Model file for the job. Use its own axes, mm. A direction names the side the tool comes from. Round coordinates to 2 decimals unless told otherwise and drop trailing zeros. Order: outer loops, then holes, each group sorted by start corner. A loop starts at its lowest first (then second) coordinate and runs counter-clockwise, first axis right, second up. Notation, with made-up numbers: (56, 30.25) -> (107, 30.25) arc R12 cw to (107, 38.25) -> close; hole circle Ø10 at (78.25, 77). An arc over 180 degrees is marked (long way). Answer as CSV lines item,"result".
Solid Edge part; units mm, degrees
sketch "Sketch1" plane through (0, 0, 0) normal (0, 0, 1) x (1, 0, 0)
  line L0 (0, 123.5) -> (0, 6.5)
  line L1 (13, 6.5) -> (13, 123.5)
  arc A0 (13, 6.5) -> (0, 6.5) centre (6.5, 6.5) cw
  arc A1 (0, 123.5) -> (13, 123.5) centre (6.5, 123.5) cw
extrude "Protrusion1" add sketch "Sketch1" along normal blind 6.5
sketch "Sketch2" plane through (6.5, 0, 0) normal (1, 0, 0) x (0, 1, 0)
  line L0 (3.5, 5.5) -> (3.5, 6.5)
  line L1 (3.5, 6.5) -> (6.5, 6.5)
  line L2 (6.5, 1) -> (6.5, 6.5)
  line L3 (3.5, 1) -> (6.5, 1)
  line L4 (3.5, 1) -> (2.6811, 3.25)
  line L5 (3.5, 5.5) -> (2.6811, 3.25)
revolve "RevolvedCutout1" cut sketch "Sketch2" angle 360 about axis through (6.5, 6.5, 1) along (0, 0, 1)
chamfer "Chaflán_38" distance 0.75 angle 45 1 edges at (6.5, 3.5, 6.5)
pattern_linear "Pattern1" count 10 spacing 13 along (0, 1, 0) of "RevolvedCutout1", "Chaflán_38"
chamfer "Chaflán_39" distance 1.5 angle 45 8 edges at (13, 65, 6.5) (6.5, 0, 6.5) (0, 65, 6.5) (6.5, 130, 6.5) (13, 65, 0) (6.5, 0, 0) (0, 65, 0) (6.5, 130, 0)
Q1. Saw through at A-A (y = 78.5). Write the cut outline in (x, z), plus the area to 3 significant figures.
Checks:
outline,"(0, 1.5) -> (1.5, 0) -> (11.5, 0) -> (13, 1.5) -> (13, 5) -> (11.5, 6.5) -> (1.5, 6.5) -> (0, 5) -> close"
area,"80.0 mm²"
Q2. Tool access for faces 4 (the conical face through (6.4, 1.2, 0.3)), 5 (the conical face through (7.669, 55.681, 5.359)), 6 (the flat face through (7, 111, 1)): list every direction of +Z, -Z, +X, -X, +Y, -Y with a clear straight run to the whole face (end or side of a thin tool).
Checks:
face 4,"-Z, -Y"
face 5,"none"
face 6,"+Z"
Q3. Mould opens along Z. For faces 1 (the flat face through (7, 72, 1)), 2 (the cylindrical face through (6.6, 0, 3.2)), 3 (the conical face through (3.927, 95.86, 5.359)) say: +Z half, -Z half, draft (parallel to the pull), parting line (faces both ways), or undercut.
Checks:
face 1,"+Z half"
face 2,"draft"
face 3,"undercut"
Q4. Flat gauge pins, fed straight in: pin 1 (7 mm diameter, centred on x = 6.5, y = 97.5, fed in from +Z); pin 2 (1.8 mm diameter, centred on x = 6, y = 44, fed in from +Z); pin 3 (3 mm diameter, centred on x = 7.5, y = 70, fed in from +Z). Where does each tip first touch, or does it go through?
Checks:
pin 1,"z = 6.25"
pin 2,"z = 1"
pin 3,"z = 6.05"
Q5. Wall check: L1, parallel to X at y = 44, z = 2; L2, parallel to X at y = 69, z = 3.5; L3, parallel to Z at x = 8, y = 32. Give the ranges that are in metal, low to high. Write a range as [from, to].
Checks:
L1,"[0, 3.49], [9.51, 13]"
L2,"[0, 3.73], [9.27, 13]"
L3,"[0, 1]"
Q6. Saw through at B-B (y = 45.5). Write the cut outline in (x, z).
Checks:
outline,"(0, 1.5) -> (1.5, 0) -> (11.5, 0) -> (13, 1.5) -> (13, 5) -> (11.5, 6.5) -> (10.25, 6.5) -> (9.5, 5.75) -> (9.5, 5.5) -> (10.32, 3.25) -> (9.5, 1) -> (3.5, 1) -> (2.68, 3.25) -> (3.5, 5.5) -> (3.5, 5.75) -> (2.75, 6.5) -> (1.5, 6.5) -> (0, 5) -> close"
